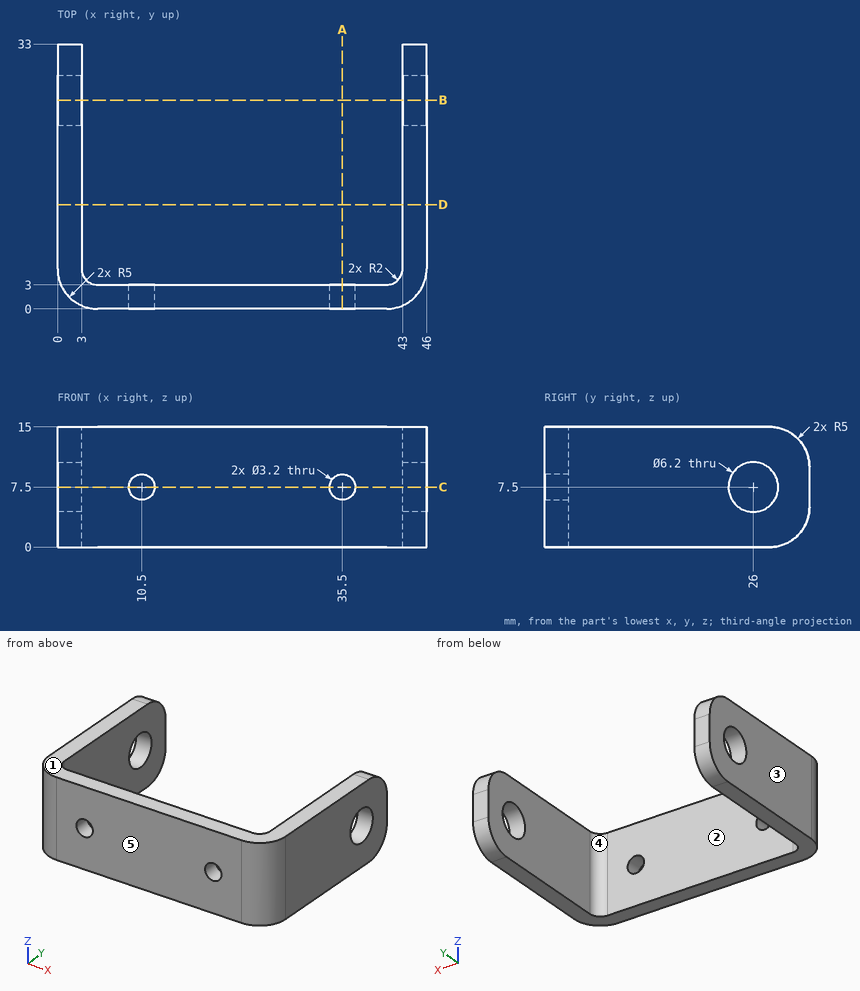
Can you work these out from the drawing? Everything is in mm from the part's minimum corner. A direction names the side the tool comes from. Round coordinates to 2 decimals unless told otherwise and drop trailing zeros. Loops run counter-clockwise (first coordinate to the right, second up) from the corner with the lowest first, then second, coordinate; pieces in that order, holes last. Notation, with made-up numbers: (-34.5, -29) -> (-11.5, -29) arc R10 ccw to (-11.5, -17) -> close; hole circle Ø3 at (-4.5, -23). An arc over 180 degrees is marked (long way). Put each result on its own line as item: value.
Q1. I want a section at B-B on y = 26. Write out the boundary of the cut face in (x, z), and give its area (3 significant figures).
Checks:
outline: (0, 0) -> (3, 0) -> (3, 4.4) -> (0, 4.4) -> close; (0, 10.6) -> (3, 10.6) -> (3, 15) -> (0, 15) -> close; (43, 0) -> (46, 0) -> (46, 4.4) -> (43, 4.4) -> close; (43, 10.6) -> (46, 10.6) -> (46, 15) -> (43, 15) -> close
area: 52.8 mm2
Q2. I want a section at C-C on z = 7.5. Write out the boundary of the cut face in (x, y), and give its area (3 significant figures).
Checks:
outline: (0, 5) arc R5 ccw to (5, 0) -> (8.9, 0) -> (8.9, 3) -> (5, 3) arc R2 cw to (3, 5) -> (3, 22.9) -> (0, 22.9) -> close; (0, 29.1) -> (3, 29.1) -> (3, 33) -> (0, 33) -> close; (12.1, 0) -> (33.9, 0) -> (33.9, 3) -> (12.1, 3) -> close; (37.1, 0) -> (41, 0) arc R5 ccw to (46, 5) -> (46, 22.9) -> (43, 22.9) -> (43, 5) arc R2 cw to (41, 3) -> (37.1, 3) -> close; (43, 29.1) -> (46, 29.1) -> (46, 33) -> (43, 33) -> close
area: 253 mm2
Q3. Please list where these lines run through material, in increasing order: line 1 (X direction, y = 27.5, z = 14.5); line 2 (X direction, y = 1.6, z = 7.5); line 3 (Y direction, x = 25, z = 12.75). Write a range as from..to.
Checks:
line 1: 0..3, 43..46
line 2: 1.33..8.9, 12.1..33.9, 37.1..44.67
line 3: 0..3
Q4. I want a section at D-D on y = 13. Write out the boundary of the cut face in (x, z), and give its area (3 significant figures).
Checks:
outline: (0, 0) -> (3, 0) -> (3, 15) -> (0, 15) -> close; (43, 0) -> (46, 0) -> (46, 15) -> (43, 15) -> close
area: 90.0 mm2
Q5. I want a section at A-A on x = 35.5. Write out the boundary of the cut face in (y, z), and give its area (3 significant figures).
Checks:
outline: (0, 0) -> (3, 0) -> (3, 5.9) -> (0, 5.9) -> close; (0, 9.1) -> (3, 9.1) -> (3, 15) -> (0, 15) -> close
area: 35.4 mm2
Q6. For pin 1 Ø3 at (x, z) = (10.5, 7.5) entering from +Y; pin 2 Ø10 at (x, y) = (17.5, 7) entering from +Z; pin 3 Ø2 at (x, z) = (33.5, 2.5) entering from +Y, each with a flat end and sliding along its axis, tell me the tip position at first contact or that it passes through.
Checks:
pin 1: through
pin 2: z = 15
pin 3: y = 3
Q7. Thinking about a two-plate mould opening in X: for the marked faces 3, 4 and 5, which applies, pulls with the +X half, pulls with the -X half, needs draft (parallel to the pull), parting line crosses it, or undercut?
Checks:
face 3: pulls with the -X half
face 4: undercut
face 5: needs draft
Q8. Which directions (+Z, -Z, +X, -X, +Y, -Y) give clear straight access to the entire face, cutting with the end or side of a thin tool? Please do the marked faces 1 and 2.
Checks:
face 1: +Z, +X, -X, +Y, -Y
face 2: +Z, -Z, +Y
